from build123d import *

# Parameters (mm, degrees)
CROQUIS1_W              = 23
CROQUIS1_H              = 23
CROQUIS1_W_2            = 19
CROQUIS1_H_2            = 19
SALIENTE_EXTRUIR1_DEPTH = 10
CROQUIS2_W              = 7
CROQUIS2_H              = 10
SALIENTE_EXTRUIR2_DEPTH = 1.5
SALIENTE_EXTRUIR3_DEPTH = 3
CROQUIS4_R              = 2
CORTAR_EXTRUIR1_DEPTH   = 4


with BuildPart() as part:
    # Croquis1 → Saliente-Extruir1 (new body)
    with BuildSketch(Plane(origin=(0, 0, 0), x_dir=(1, 0, 0), z_dir=(0, 1, 0))):
        Rectangle(CROQUIS1_W, CROQUIS1_H)
        Rectangle(CROQUIS1_W_2, CROQUIS1_H_2, mode=Mode.SUBTRACT)
    extrude(amount=SALIENTE_EXTRUIR1_DEPTH)

    # Croquis2 → Saliente-Extruir2 (add, symmetric)
    with BuildSketch(Plane(origin=(0, 0, 0), x_dir=(0, 0, -1), z_dir=(1, 0, 0))):
        with Locations((15, 5)):
            Rectangle(CROQUIS2_W, CROQUIS2_H)
    saliente_extruir2 = extrude(amount=SALIENTE_EXTRUIR2_DEPTH, both=True)

    # Croquis3 → Saliente-Extruir3 (add)
    with BuildSketch(Plane(origin=(0, 0, -18.5), x_dir=(-1, 0, 0), z_dir=(0, 0, -1))):
        Polygon((-9, 10), (-11.5, 7.5), (-11.5, 2.5), (-9, 0), (1.5, 0), (1.5, 10), align=None)
    saliente_extruir3 = extrude(amount=SALIENTE_EXTRUIR3_DEPTH)

    # Croquis4 → Cortar-Extruir1 (cut)
    with BuildSketch(Plane(origin=(0, 0, -21.5), x_dir=(-1, 0, 0), z_dir=(0, 0, -1))):
        with Locations((-6.5, 5)):
            Circle(CROQUIS4_R)
    cortar_extruir1 = extrude(amount=-CORTAR_EXTRUIR1_DEPTH, mode=Mode.SUBTRACT)

    # Simetría1: Saliente-Extruir2, Saliente-Extruir3, Cortar-Extruir1 across plane
    add(saliente_extruir2.mirror(Plane.XY))
    add(saliente_extruir3.mirror(Plane.XY))
    add(cortar_extruir1.mirror(Plane.XY), mode=Mode.SUBTRACT)


solid = part.part
Here's how the part is built. I have some questions about the finished solid (model axes, mm). A direction names the side the tool comes from. Coordinates: 2 decimals unless noted, no trailing zeros. Order: outer loops, then holes, each group sorted by start corner. A loop starts at its lowest first (then second) coordinate and runs counter-clockwise, first axis right, second up. Notation, with made-up numbers: M 58.25,-9 L 65.25,-9 A18 cw 65.25,26 Z; hole C 49,82.5 d1. An arc over 180 degrees is marked long. Answer as CSV lines item,"result". Start each with the question number.
1. I want a section at A-A, the plane y = 5. Write out the boundary of the cut face in (x, z), and give its area (3 significant figures).
2. I want a section at D-D, the plane y = 9.25. Write out the boundary of the cut face in (x, z).
3. For pin 1 (3 mm diameter, centred on x = -7, y = 4, fed in from -Z); pin 2 (5 mm diameter, centred on x = -5.5, y = 9, fed in from +Z); pin 3 (2 mm diameter, centred on y = 7.5, z = -14.5, fed in from +X), each with a flat end and sliding along its axis, tell me the tip position at first contact or that it passes through.
4. We'd pull the mould along Y, two halves only. Please class faces 1 (the flat face through (10, 9, -20)), 2 (the cylindrical face through (8.498, 5.088, -20.021)), 3 (the flat face through (1, 0, -10)), 4 (the flat face through (4, 5, -21.5)): released by +Y, released by -Y, zero draft, split by the parting line, or undercut.
5. I need wall thicknesses on line 1 (Z direction, x = 10.5, y = 4.75); line 2 (Z direction, x = 4.5, y = 6.5); line 3 (X direction, y = 0.75, z = 6). Which ranges of each line are inside material? Lowest first, please. Write a range as [from, to].
6. I want a section at C-C, the plane z = 4. Write out the boundary of the cut face in (x, y), and give its area (3 significant figures).
7. I want a section at B-B, the plane x = -9. Write out the boundary of the cut face in (y, z).
8. On a 3-axis mill with a long thin cutter (end or side, diameter ignored), from which of +Z, -Z, +X, -X, +Y, -Y can I reach the whole of each face in a straight line? I mean faces 5 (the flat face through (-1.5, 5, -16)), 6 (the flat face through (-9.5, 5, 0)), 7 (the flat face through (-7, 5, 11.5)). Say none if no direction works.
Recorded:
1,outline,"M -11.5,-11.5 L -1.5,-11.5 L -1.5,-21.5 L 4.5,-21.5 L 4.5,-18.5 L 1.5,-18.5 L 1.5,-11.5 L 11.5,-11.5 L 11.5,11.5 L 1.5,11.5 L 1.5,18.5 L 4.5,18.5 L 4.5,21.5 L -1.5,21.5 L -1.5,11.5 L -11.5,11.5 Z; M 8.5,-21.5 L 11.5,-21.5 L 11.5,-18.5 L 8.5,-18.5 Z; M 8.5,18.5 L 11.5,18.5 L 11.5,21.5 L 8.5,21.5 Z; hole M -9.5,-9.5 L 9.5,-9.5 L 9.5,9.5 L -9.5,9.5 Z"
1,area,"264 mm2"
2,outline,"M -11.5,-11.5 L -1.5,-11.5 L -1.5,-21.5 L 9.75,-21.5 L 9.75,-18.5 L 1.5,-18.5 L 1.5,-11.5 L 11.5,-11.5 L 11.5,11.5 L 1.5,11.5 L 1.5,18.5 L 9.75,18.5 L 9.75,21.5 L -1.5,21.5 L -1.5,11.5 L -11.5,11.5 Z; hole M -9.5,-9.5 L 9.5,-9.5 L 9.5,9.5 L -9.5,9.5 Z"
3,pin 1,"stops at z = -11.5"
3,pin 2,"stops at z = 11.5"
3,pin 3,"stops at x = 1.5"
4,face 1,"released by +Y"
4,face 2,"undercut"
4,face 3,"released by -Y"
4,face 4,"zero draft"
5,line 1,"z = [-21.5, -18.5], [-11.5, 11.5], [18.5, 21.5]"
5,line 2,"z = [-21.5, -18.5], [-11.5, -9.5], [9.5, 11.5], [18.5, 21.5]"
5,line 3,"x = [-11.5, -9.5], [9.5, 11.5]"
6,outline,"M -11.5,0 L -9.5,0 L -9.5,10 L -11.5,10 Z; M 9.5,0 L 11.5,0 L 11.5,10 L 9.5,10 Z"
6,area,"40.0 mm2"
7,outline,"M 0,-11.5 L 10,-11.5 L 10,-9.5 L 0,-9.5 Z; M 0,9.5 L 10,9.5 L 10,11.5 L 0,11.5 Z"
8,face 5,"-Z, -X, +Y, -Y"
8,face 6,"+Y, -Y"
8,face 7,"+Z, -X, +Y, -Y"
